from build123d import *

# Parameters (mm, degrees)
F0_W     = 58.45416
F0_H     = 41.958041
F1_DEPTH = 10
F2_R     = 5.628683
F3_DEPTH = 10.001


with BuildPart() as f1:
    # F0 (on Front) → F1 (new body)
    with BuildSketch(Plane.XZ):
        with Locations((29.22708, 20.979021)):
            Rectangle(F0_W, F0_H)
    extrude(amount=F1_DEPTH)

    # F2 (on face) → F3 (cut, through all)
    with BuildSketch(Plane.XZ.offset(10)):
        with Locations((11.372562, 31.127132)):
            Circle(F2_R)
    extrude(amount=-F3_DEPTH, mode=Mode.SUBTRACT)

    # F4 (on face) → F5 (revolve)
    with BuildSketch(Plane.XZ.offset(10)):
        Polygon((49.627889, 25.171686), (34.761366, 31.748787), (15.927874, 20.762276), (35.032336, 13.681269), (23.995256, 9.382639), (54.431368, 5.763666), align=None)
    revolve(axis=Axis((58.45416, -10, 20.979021), (0, 0, -1)))


solid = f1.part
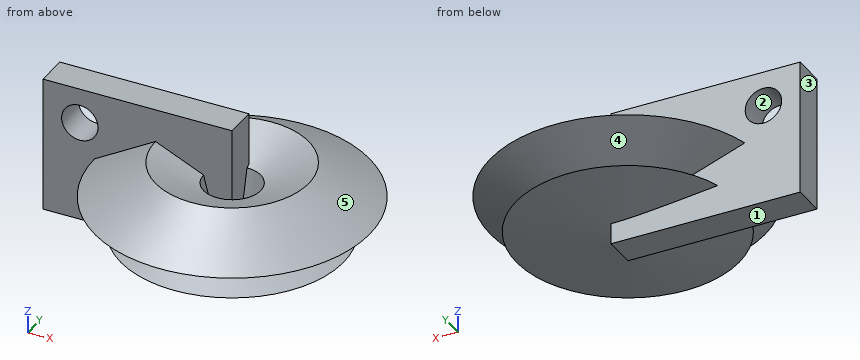
Can you work these out from the model? Positions are in its coordinate system, mm. Face numbers are marked on the shaded views. A direction names the side the tool comes from. Coordinates: 2 decimals unless noted, no trailing zeros. Write each loop counter-clockwise with the first axis right and the second up, starting at its lowest first coordinate (ties: lowest second). Pieces come first, ordered by that corner, then holes. Notation, with made-up numbers: (41.5, -22.5) -> (86.5, -22.5) arc R18 cw to (86.5, 11.5) -> close; hole circle Ø10 at (47.25, 18). An arc over 180 degrees is marked (long way). Write each question's results on one line, items separated by ' | '. Start each with the question number.
Item 1: On a 3-axis mill with a long thin cutter (end or side, diameter ignored), from which of +Z, -Z, +X, -X, +Y, -Y can I reach the whole of each face in a straight line? I mean the marked faces 4 and 5. Say none if no direction works.
Item 2: If we section it at A-A, the plane z = 27: Write out the boundary of the cut face in (x, y), and give its area (3 significant figures).
Item 3: If we section it at B-B, the plane x = 14.5: Write out the boundary of the cut face in (y, z), and give its area (3 significant figures).
Item 4: If we section it at C-C, the plane z = 16: Write out the boundary of the cut face in (x, y), and give its area (3 significant figures).
Item 5: I'm going to push flat-ended pins straight in: P1, Ø8, axis at y = -5.5, z = 31, coming from the +X side; P2, Ø1.5, axis at x = 58, y = 16.5, coming from the +Z side; P3, Ø3, axis at x = 54, z = 35.5, coming from the +Y side. Where does each tip first touch, or does it pass through?
Item 6: Thinking about a two-plate mould opening in Z: for the marked faces 1, 2 and 3, which applies, released by +Z, released by -Z, zero draft, split by the parting line, or undercut?
Item 7: Please list where these lines run through material, in increasing order: probe 1 along X at (y, z) = (-7, 28.5); probe 2 along Y at (x, z) = (17, 34.5); probe 3 along Y at (x, z) = (59, 23.5).
Answer block:
1) face 4: none | face 5: +Z
2) outline: (0, -10) -> (7.55, -10) -> (7.55, 0) -> (0, 0) -> close; (15.2, -10) -> (26.62, -10) arc R31.83 ccw (long way) to (28.23, 0) -> (15.2, 0) -> close; hole (45.5, -10) arc R12.96 ccw (long way) to (50.21, 0) -> (58.45, 0) -> (58.45, -10) -> close | area: 2,970 mm²
3) outline: (-10, 0) -> (0, 0) -> (0, 26.45) -> (-10, 26.45) -> close; (-10, 35.81) -> (0, 35.81) -> (0, 41.96) -> (-10, 41.96) -> close | area: 326 mm²
4) outline: (0, -10) -> (28.78, -10) arc R29.68 ccw (long way) to (30.51, 0) -> (0, 0) -> close; hole (51.9, -10) arc R6.56 ccw (long way) to (58.45, -3.44) -> (58.45, -10) -> close | area: 2,960 mm²
5) P1: x = 89.99 | P2: z = 30.55 | P3: y = 0
6) face 1: released by -Z | face 2: undercut | face 3: zero draft
7) probe 1: 0 to 6.39, 16.35 to 58.45, 74.53 to 87.56 | probe 2: -10 to 0 | probe 3: -47.83 to -18.39, -1.61 to 27.83
